Can you work these out from the model? Positions are in its coordinate system, mm. A direction names the side the tool comes from. Coordinates: 2 decimals unless noted, no trailing zeros. Order: outer loops, then holes, each group sorted by start corner. A loop starts at its lowest first (then second) coordinate and runs counter-clockwise, first axis right, second up. Notation, with made-up numbers: (54, 55) -> (80, 55) arc R14 ccw to (80, 66) -> close; hole circle Ø5 at (59.5, 19). An arc over 180 degrees is marked (long way). Answer in a Markdown table with one row per item.
```python
from build123d import *

# Parameters (mm, degrees)
SKETCH_R        = 2.8
SKETCH_R_2      = 19.914493
PAD_DEPTH       = 20
SKETCH001_W     = 57.5
SKETCH001_H     = 58
POCKET_DEPTH    = 12
POCKET001_DEPTH = 308.202319
FILLET_R        = 4
FILLET001_R     = 1
CHAMFER_SIZE    = 1
CHAMFER001_SIZE = 1


with BuildPart() as part:
    # Sketch → Pad (new body)
    with BuildSketch(Plane.XZ):
        Polygon((33, -18), (33, 29), (-33, 29), (-33, -18), (-63, -18), (-63, -38), (63, -38), (63, -18), align=None)
        with Locations((-23.57, -23.57)):
            Circle(SKETCH_R, mode=Mode.SUBTRACT)
        with Locations((23.57, -23.57)):
            Circle(SKETCH_R, mode=Mode.SUBTRACT)
        with Locations((-23.57, 23.57)):
            Circle(SKETCH_R, mode=Mode.SUBTRACT)
        Circle(SKETCH_R_2, mode=Mode.SUBTRACT)
        with Locations((23.57, 23.57)):
            Circle(SKETCH_R, mode=Mode.SUBTRACT)
    extrude(amount=PAD_DEPTH)

    # Sketch001 (on Face14 of Pad) → Pocket (cut)
    with BuildSketch(Plane(origin=(0, 0, 0), x_dir=(1, 0, 0), z_dir=(0, 1, 0))):
        Rectangle(SKETCH001_W, SKETCH001_H)
    extrude(amount=-POCKET_DEPTH, mode=Mode.SUBTRACT)

    # Sketch002 (on Face2 of Pocket) → Pocket001 (cut, through all)
    with BuildSketch(Plane(origin=(0, 0, -18), x_dir=(-1, 0, 0), z_dir=(0, 0, 1))):
        with BuildLine():
            ThreePointArc((-55.5, 12.5), (-58, 10), (-55.5, 7.5))
            Line((-55.5, 7.5), (-40.5, 7.5))
            ThreePointArc((-40.5, 7.5), (-38, 10), (-40.5, 12.5))
            Line((-55.5, 12.5), (-40.5, 12.5))
        make_face()
    pocket001 = extrude(amount=-POCKET001_DEPTH, mode=Mode.SUBTRACT)

    # Mirrored: Pocket001 across Sketch002 V_Axis
    add(pocket001.mirror(Plane(origin=(0, 0, -18), x_dir=(0, 0, 1), z_dir=(-1, 0, 0))), mode=Mode.SUBTRACT)

    # Fillet
    fillet_edges = [part.edges().sort_by_distance(p)[0] for p in [
        (33, -10, -18),
        (-33, -10, -18),
    ]]
    fillet(fillet_edges, radius=FILLET_R)

    # Fillet001
    fillet001_edges = [part.edges().sort_by_distance(p)[0] for p in [
        (33, 0, 7.5),
        (-33, 0, 7.5),
        (33, -20, 7.5),
        (-33, -20, 7.5),
        (63, -10, -18),
        (-63, -10, -18),
        (-63, 0, -28),
        (-63, -20, -28),
        (63, 0, -28),
        (63, -20, -28),
    ]]
    fillet(fillet001_edges, radius=FILLET001_R)

    # Chamfer
    chamfer_edges = [part.edges().sort_by_distance(p)[0] for p in [
        (28.75, -6, -29),
        (-28.75, -6, -29),
    ]]
    chamfer(chamfer_edges, length=CHAMFER_SIZE)

    # Chamfer001
    chamfer001_edges = [part.edges().sort_by_distance(p)[0] for p in [
        (-19.914493, -12, 0),
    ]]
    chamfer(chamfer001_edges, length=CHAMFER001_SIZE)


solid = part.part
```
(1) Suppose I cut it at A-A (x = -51). Please give me the cut outline in (y, z).
Response values:
| item | result |
|---|---|
| outline | (-20, -38) -> (-12.5, -38) -> (-12.5, -18) -> (-19, -18) arc R1 ccw to (-20, -19) -> close; (-7.5, -38) -> (0, -38) -> (0, -19) arc R1 ccw to (-1, -18) -> (-7.5, -18) -> close |
(2) We'd pull the mould along Z, two halves only. Please class faces 6 (the flat face through (0, -6, -29)), 7 (the flat face through (28.75, -6, 1)), 8 (the cylindrical face through (-22.06, -15.94, -21.21)): +Z half, -Z half, draft (parallel to the pull), parting line (faces both ways), or undercut.
Response values:
| item | result |
|---|---|
| face 6 | +Z half |
| face 7 | draft |
| face 8 | undercut |
(3) Will these pins go through, and if not, where does the flat tip stop? pin 1 Ø7.5 at (x, z) = (-23.57, -23.57) entering from +Y; pin 2 Ø9.5 at (y, z) = (-8.5, 5) entering from -X; pin 3 Ø9.5 at (y, z) = (-7.5, 9.5) entering from +X.
Response values:
| item | result |
|---|---|
| pin 1 | y = -12 |
| pin 2 | x = -33 |
| pin 3 | x = 33 |
(4) On a 3-axis mill with a long thin cutter (end or side, diameter ignored), from which of +Z, -Z, +X, -X, +Y, -Y can I reach the whole of each face in a straight line? I mean faces 1 (the cylindrical face through (-38, -10, -28)), 2 (the flat face through (50, -14, -18)), 3 (the cylindrical face through (18.995, -16.451, 5.982)), 4 (the flat face through (-28.75, -6, 1)), 5 (the flat face through (-49, -14, -18)). Say none if no direction works.
Response values:
| item | result |
|---|---|
| face 1 | +Z, -Z |
| face 2 | +Z, +X, +Y, -Y |
| face 3 | +Y, -Y |
| face 4 | +Z, +Y |
| face 5 | +Z, -X, +Y, -Y |
(5) Suppose I cut it at C-C (z = -23.57). Please give me the cut outline in (x, y).
Response values:
| item | result |
|---|---|
| outline | (-63, -19) arc R1 ccw to (-62, -20) -> (-26.37, -20) -> (-26.37, -12) -> (-28.75, -12) -> (-28.75, 0) -> (-62, 0) arc R1 ccw to (-63, -1) -> close; (-20.77, -20) -> (20.77, -20) -> (20.77, -12) -> (-20.77, -12) -> close; (26.37, -20) -> (62, -20) arc R1 ccw to (63, -19) -> (63, -1) arc R1 ccw to (62, 0) -> (28.75, 0) -> (28.75, -12) -> (26.37, -12) -> close; hole (-55.5, -12.5) -> (-40.5, -12.5) arc R2.5 ccw to (-40.5, -7.5) -> (-55.5, -7.5) arc R2.5 ccw to start; hole (40.5, -12.5) -> (55.5, -12.5) arc R2.5 ccw to (55.5, -7.5) -> (40.5, -7.5) arc R2.5 ccw to start |
(6) I need wall thicknesses on line 1 (Z direction, x = -23.57, y = -14); line 2 (X direction, y = -16.5, z = 23.57); line 3 (X direction, y = -15.5, z = -23.57). Which ranges of each line are inside material? Lowest first, please. Write a range as [from, to].
Response values:
| item | result |
|---|---|
| line 1 | [-38, -26.37], [-20.77, 20.77], [26.37, 29] |
| line 2 | [-33, -26.37], [-20.77, 20.77], [26.37, 33] |
| line 3 | [-63, -26.37], [-20.77, 20.77], [26.37, 63] |
(7) Suppose I cut it at D-D (z = 23.57). Please give me the cut outline in (x, y), and give its area (3 significant figures).
Response values:
| item | result |
|---|---|
| outline | (-33, -19) arc R1 ccw to (-32, -20) -> (-26.37, -20) -> (-26.37, -12) -> (-28.75, -12) -> (-28.75, 0) -> (-32, 0) arc R1 ccw to (-33, -1) -> close; (-20.77, -20) -> (20.77, -20) -> (20.77, -12) -> (-20.77, -12) -> close; (26.37, -20) -> (32, -20) arc R1 ccw to (33, -19) -> (33, -1) arc R1 ccw to (32, 0) -> (28.75, 0) -> (28.75, -12) -> (26.37, -12) -> close |
| area | 540 mm2 |
(8) Suppose I cut it at B-B (y = -10). Please give me the cut outline in (x, z), and give its area (3 significant figures).
Response values:
| item | result |
|---|---|
| outline | (-63, -38) -> (-58, -38) -> (-58, -18) -> (-62, -18) arc R1 ccw to (-63, -19) -> close; (-38, -38) -> (38, -38) -> (38, -18) -> (37, -18) arc R4 cw to (33, -14) -> (33, 29) -> (28.75, 29) -> (28.75, -28) -> (27.75, -29) -> (-27.75, -29) -> (-28.75, -28) -> (-28.75, 29) -> (-33, 29) -> (-33, -14) arc R4 cw to (-37, -18) -> (-38, -18) -> close; (58, -38) -> (63, -38) -> (63, -19) arc R1 ccw to (62, -18) -> (58, -18) -> close |
| area | 1,490 mm2 |
